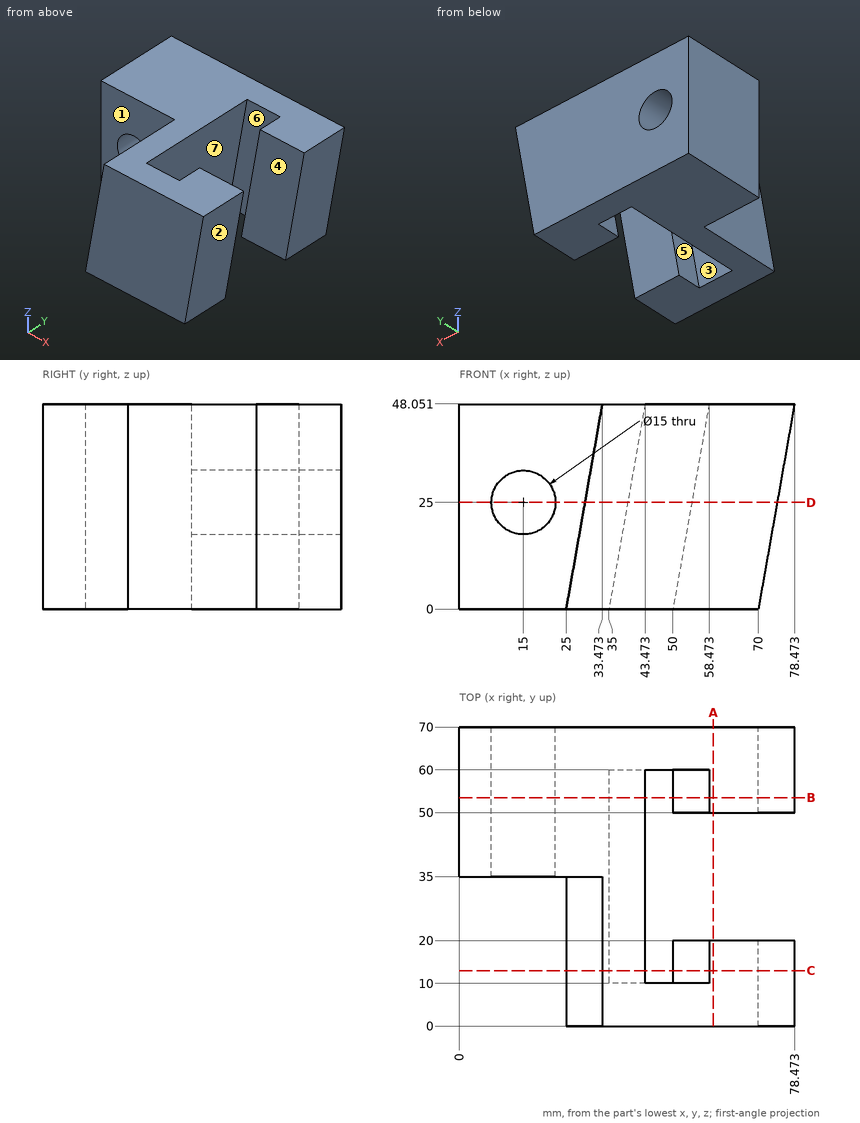
Answer from the drawing. Dimensions are ordinates in mm from the lowest x, y and z of the part. A direction names the side the tool comes from. Coordinates: 2 decimals unless noted, no trailing zeros. Loops run counter-clockwise (first coordinate to the right, second up) from the corner with the lowest first, then second, coordinate; pieces in that order, holes last. Notation, with made-up numbers: (47.25, 67) -> (95.25, 67) arc R23 cw to (95.25, 81) -> close; hole circle Ø10 at (-34.5, -27). An arc over 180 degrees is marked (long way). Answer in a Markdown table with one row per item.
Item 1: For the marked faces 4, 5, 6 and 7, determine the directions among +Z, -Z, +X, -X, +Y, -Y from which every point of the face is accessible in a straight line to the end or side of a thin tool.
Returned:
| item | result |
|---|---|
| face 4 | +Z, -Z, +X |
| face 5 | +Z |
| face 6 | none |
| face 7 | -Z |
Item 2: A cutting plane is placed at A-A on x = 59.5. Determine the outline of the cut face in (y, z).
Returned:
| item | result |
|---|---|
| outline | (0, 0) -> (20, 0) -> (20, 48.05) -> (0, 48.05) -> close; (50, 0) -> (70, 0) -> (70, 48.05) -> (50, 48.05) -> close |
Item 3: A cutting plane is placed at B-B on y = 53.5. Determine the outline of the cut face in (x, z).
Returned:
| item | result |
|---|---|
| outline | (0, 0) -> (35, 0) -> (43.47, 48.05) -> (0, 48.05) -> close; (50, 0) -> (70, 0) -> (78.47, 48.05) -> (58.47, 48.05) -> close; hole circle Ø15 at (15, 25) |
Item 4: A cutting plane is placed at D-D on z = 25. Determine the outline of the cut face in (x, y).
Returned:
| item | result |
|---|---|
| outline | (0, 35) -> (7.5, 35) -> (7.5, 70) -> (0, 70) -> close; (22.5, 35) -> (29.41, 35) -> (29.41, 0) -> (74.41, 0) -> (74.41, 20) -> (54.41, 20) -> (54.41, 10) -> (39.41, 10) -> (39.41, 60) -> (54.41, 60) -> (54.41, 50) -> (74.41, 50) -> (74.41, 70) -> (22.5, 70) -> close |
Item 5: For a pull along X with two mould halves and no side action, classify the marked faces 1, 2 and 3 as released by +X, released by -X, zero draft, split by the parting line, or undercut.
Returned:
| item | result |
|---|---|
| face 1 | zero draft |
| face 2 | released by +X |
| face 3 | undercut |
Item 6: A cutting plane is placed at C-C on y = 13. Determine the outline of the cut face in (x, z), plus the area to 3 significant figures.
Returned:
| item | result |
|---|---|
| outline | (25, 0) -> (35, 0) -> (43.47, 48.05) -> (33.47, 48.05) -> close; (50, 0) -> (70, 0) -> (78.47, 48.05) -> (58.47, 48.05) -> close |
| area | 1,440 mm^2 |
Item 7: Straight lines are drawn through the part: line 1 along Y through (x, z) = (56, 19.5); line 2 along Y through (x, z) = (51.5, 27); line 3 along X through (y, z) = (58.5, 25). For each, find the intervals that lie inside material, in ascending order. Write a range as [from, to].
Returned:
| item | result |
|---|---|
| line 1 | y = [0, 20], [50, 70] |
| line 2 | y = [0, 10], [60, 70] |
| line 3 | x = [0, 7.5], [22.5, 39.41], [54.41, 74.41] |
Item 8: Each of these flat-tipped pins is pushed along its axis until it touches: P1, Ø6, axis at y = 46, z = 28, coming from the +X side; P2, Ø10, axis at y = 42.5, z = 6, coming from the +X side; P3, Ø3, axis at x = 27, z = 28, coming from the -Y side; P4, Ø5, axis at x = 52.5, y = 24.5, coming from the +Z side. Where does it stop, or does it pass through?
Returned:
| item | result |
|---|---|
| P1 | stops at x = 40.47 |
| P2 | stops at x = 36.94 |
| P3 | stops at y = 35 |
| P4 | passes through |
